```python
from build123d import *

# Parameters (mm, degrees)
BOSS_EXTRUDE1_DEPTH = 2.032
FILLET1_R           = 3
FILLET2_R           = 2
SKETCH4_R           = 1.5875
CUT_EXTRUDE1_DEPTH  = 136.528598113


with BuildPart() as part:
    # Sketch3 → Boss-Extrude1 (new body)
    with BuildSketch(Plane.XY):
        with BuildLine():
            ThreePointArc((4.075, 10.775), (9.233659082, 17.295296632), (16.76582632, 13.775))
            Line((16.76582632, 13.775), (27.78417368, 13.775))
            ThreePointArc((27.78417368, 13.775), (33.775, 17.475), (39.76582632, 13.775))
            Line((39.76582632, 13.775), (50.78417368, 13.775))
            ThreePointArc((50.78417368, 13.775), (56.775, 17.475), (62.76582632, 13.775))
            Line((62.76582632, 13.775), (73.78417368, 13.775))
            ThreePointArc((73.78417368, 13.775), (79.775, 17.475), (85.76582632, 13.775))
            Line((85.76582632, 13.775), (96.78417368, 13.775))
            ThreePointArc((96.78417368, 13.775), (102.775, 17.475), (108.76582632, 13.775))
            Line((108.76582632, 13.775), (119.78417368, 13.775))
            ThreePointArc((119.78417368, 13.775), (127.316340918, 17.295296632), (132.475, 10.775))
            Line((132.475, 10.775), (132.475, 28.535))
            Line((132.475, 28.535), (4.075, 28.535))
            Line((4.075, 28.535), (4.075, 10.775))
        make_face()
    extrude(amount=BOSS_EXTRUDE1_DEPTH)

    # Fillet1
    fillet1_edges = [part.edges().sort_by_distance(p)[0] for p in [
        (4.075, 28.535, 1.016),
        (132.475, 28.535, 1.016),
    ]]
    fillet(fillet1_edges, radius=FILLET1_R)

    # Fillet2
    fillet2_edges = [part.edges().sort_by_distance(p)[0] for p in [
        (119.78417368, 13.775, 1.016),
    ]]
    fillet(fillet2_edges, radius=FILLET2_R)
    fillet2_2_edges = [part.edges().sort_by_distance(p)[0] for p in [
        (108.76582632, 13.775, 1.016),
    ]]
    fillet(fillet2_2_edges, radius=FILLET2_R)
    fillet2_3_edges = [part.edges().sort_by_distance(p)[0] for p in [
        (96.78417368, 13.775, 1.016),
    ]]
    fillet(fillet2_3_edges, radius=FILLET2_R)
    fillet2_4_edges = [part.edges().sort_by_distance(p)[0] for p in [
        (4.075, 10.775, 1.016),
    ]]
    fillet(fillet2_4_edges, radius=FILLET2_R)
    fillet2_5_edges = [part.edges().sort_by_distance(p)[0] for p in [
        (85.76582632, 13.775, 1.016),
    ]]
    fillet(fillet2_5_edges, radius=FILLET2_R)
    fillet2_6_edges = [part.edges().sort_by_distance(p)[0] for p in [
        (16.76582632, 13.775, 1.016),
    ]]
    fillet(fillet2_6_edges, radius=FILLET2_R)
    fillet2_7_edges = [part.edges().sort_by_distance(p)[0] for p in [
        (73.78417368, 13.775, 1.016),
    ]]
    fillet(fillet2_7_edges, radius=FILLET2_R)
    fillet2_8_edges = [part.edges().sort_by_distance(p)[0] for p in [
        (27.78417368, 13.775, 1.016),
    ]]
    fillet(fillet2_8_edges, radius=FILLET2_R)
    fillet2_9_edges = [part.edges().sort_by_distance(p)[0] for p in [
        (62.76582632, 13.775, 1.016),
    ]]
    fillet(fillet2_9_edges, radius=FILLET2_R)
    fillet2_10_edges = [part.edges().sort_by_distance(p)[0] for p in [
        (39.76582632, 13.775, 1.016),
    ]]
    fillet(fillet2_10_edges, radius=FILLET2_R)
    fillet2_11_edges = [part.edges().sort_by_distance(p)[0] for p in [
        (50.78417368, 13.775, 1.016),
    ]]
    fillet(fillet2_11_edges, radius=FILLET2_R)
    fillet2_12_edges = [part.edges().sort_by_distance(p)[0] for p in [
        (132.475, 10.775, 1.016),
    ]]
    fillet(fillet2_12_edges, radius=FILLET2_R)

    # Sketch4 → Cut-Extrude1 (cut, through all)
    with BuildSketch(Plane(origin=(0, 0, 0), x_dir=(-1, 0, 0), z_dir=(0, 0, -1))):
        with Locations((-22.275, 22.185)):
            Circle(SKETCH4_R)
        with Locations((-68.275, 22.185)):
            Circle(SKETCH4_R)
        with Locations((-114.275, 22.185)):
            Circle(SKETCH4_R)
    extrude(amount=-CUT_EXTRUDE1_DEPTH, mode=Mode.SUBTRACT)


solid = part.part
```
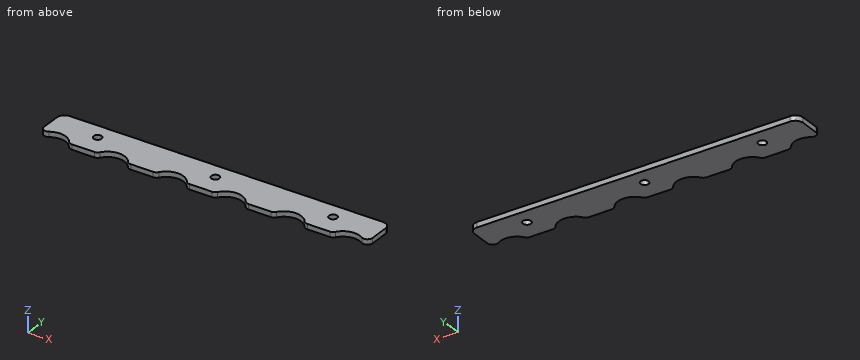
The listing builds one solid part. Answer for the finished solid, in the listing's coordinates (mm). Give positions to 0.01 mm unless a question says otherwise; leave off trailing zeros. Loops run counter-clockwise (first coordinate to the right, second up) from the corner with the lowest first, then second, coordinate; pieces in that order, holes last. Notation, with made-up numbers: M 45.25,-6 L 103.25,-6 A26 cw 103.25,13 Z; hole C -1,26.5 d6. An arc over 180 degrees is marked long. One line per item, written item: value.
1. Each of these flat-tipped pins is pushed along its axis until it touches: P1, Ø2, axis at x = 18.5, y = 16.5, coming from the -Z side; P2, Ø3, axis at x = 114.275, y = 22.185, coming from the -Z side. Where does it stop, or does it pass through?
Found:
P1: z = 0
P2: through
2. Find the intervals of material crossed by probe 1 along X at (y, z) = (22.25, 1.7) (3 decimals); probe 2 along X at (y, z) = (22.5, 0.85) (3 decimals); probe 3 along X at (y, z) = (14.5, 0.3), in increasing order.
Found:
probe 1: 4.075 to 20.689, 23.861 to 66.689, 69.861 to 112.689, 115.861 to 132.475
probe 2: 4.075 to 20.719, 23.831 to 66.719, 69.831 to 112.719, 115.831 to 132.475
probe 3: 16.35 to 28.2, 39.35 to 51.2, 62.35 to 74.2, 85.35 to 97.2, 108.35 to 120.2
3. Section C-C on x = 13 is taken. Determine the outline of the cut face in (y, z) (3 decimals), plus the area to 3 significant figures.
Found:
outline: M 17.095,0 L 28.535,0 L 28.535,2.032 L 17.095,2.032 Z
area: 23.2 mm^2
4. Section A-A on x = 114.5 is taken. Determine the outline of the cut face in (y, z) (3 decimals).
Found:
outline: M 13.775,0 L 20.614,0 L 20.614,2.032 L 13.775,2.032 Z; M 23.756,0 L 28.535,0 L 28.535,2.032 L 23.756,2.032 Z
5. Section B-B on z = 0.5 is taken. State how many separate pieces and enclosed holes the cut face has, plus the area to 3 significant figures.
Found:
separate pieces: 1
enclosed holes: 3
area: 1,670 mm^2
